Here's the drawing with two shaded views (mm, measured from the low corner). I have some questions. Coordinates: 2 decimals unless noted, no trailing zeros. Write each loop counter-clockwise with the first axis right and the second up, starting at its lowest first coordinate (ties: lowest second). Pieces come first, ordered by that corner, then holes. Notation, with made-up numbers: (9, -26.75) -> (23, -26.75) arc R32 ccw to (23, 3.25) -> close; hole circle Ø11 at (51.25, -22.5). An arc over 180 degrees is marked (long way). Put each result on its own line as item: value. Start each with the question number.
Item 1: I want a section at B-B, the plane y = 8.5. List the corners of the cut face in (x, z) for me.
Item 2: I want a section at C-C, the plane z = 1.5. List the corners of the cut face in (x, y) for me.
Item 3: I need wall thicknesses on line 1 (X direction, y = 9, z = 1.2); line 2 (Y direction, x = 35, z = 1.45); line 3 (Y direction, x = 14, z = 0.25). Which ranges of each line are inside material? Lowest first, please. Write a range as [from, to].
Item 4: I want a section at A-A, the plane x = 35. List the corners of the cut face in (y, z) for me.
Item 5: I want a section at D-D, the plane x = 24.5. List the corners of the cut face in (y, z) for me, then the cut area to 3 significant figures.
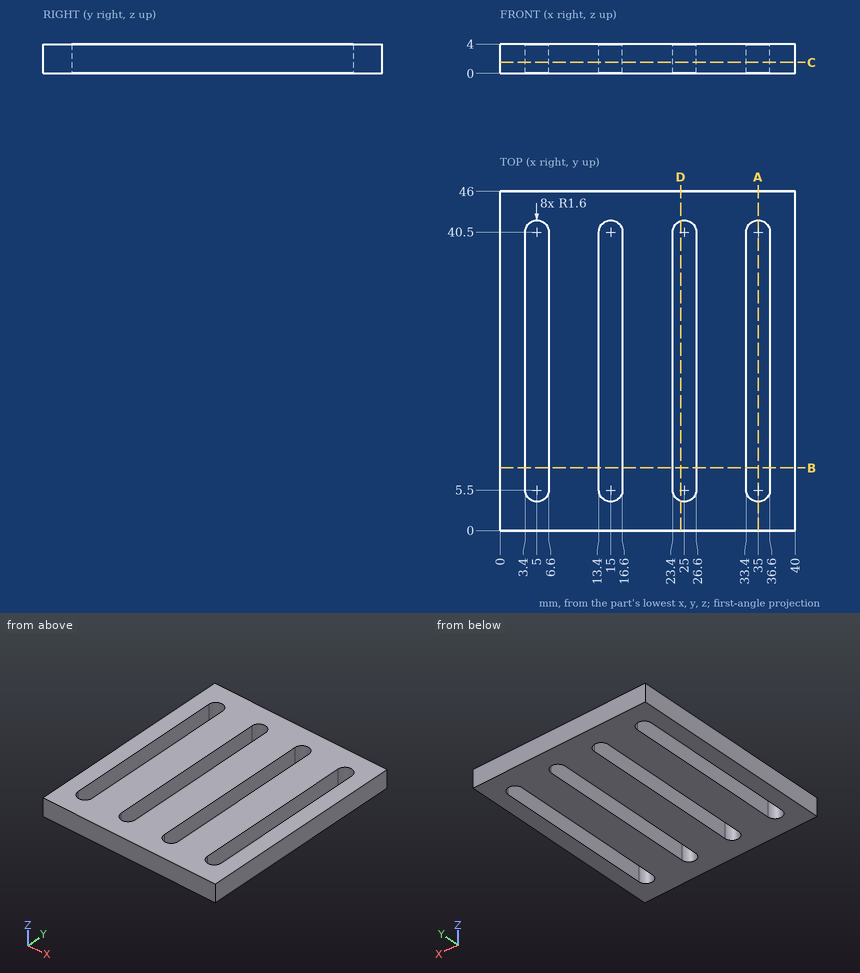
Calculated:
1. outline: (0, 0) -> (3.4, 0) -> (3.4, 4) -> (0, 4) -> close; (6.6, 0) -> (13.4, 0) -> (13.4, 4) -> (6.6, 4) -> close; (16.6, 0) -> (23.4, 0) -> (23.4, 4) -> (16.6, 4) -> close; (26.6, 0) -> (33.4, 0) -> (33.4, 4) -> (26.6, 4) -> close; (36.6, 0) -> (40, 0) -> (40, 4) -> (36.6, 4) -> close
2. outline: (0, 0) -> (40, 0) -> (40, 46) -> (0, 46) -> close; hole (3.4, 5.5) arc R1.6 ccw to (6.6, 5.5) -> (6.6, 40.5) arc R1.6 ccw to (3.4, 40.5) -> close; hole (13.4, 5.5) arc R1.6 ccw to (16.6, 5.5) -> (16.6, 40.5) arc R1.6 ccw to (13.4, 40.5) -> close; hole (23.4, 5.5) arc R1.6 ccw to (26.6, 5.5) -> (26.6, 40.5) arc R1.6 ccw to (23.4, 40.5) -> close; hole (33.4, 5.5) arc R1.6 ccw to (36.6, 5.5) -> (36.6, 40.5) arc R1.6 ccw to (33.4, 40.5) -> close
3. line 1: x = [0, 3.4], [6.6, 13.4], [16.6, 23.4], [26.6, 33.4], [36.6, 40]
3. line 2: y = [0, 3.9], [42.1, 46]
3. line 3: y = [0, 4.25], [41.75, 46]
4. outline: (0, 0) -> (3.9, 0) -> (3.9, 4) -> (0, 4) -> close; (42.1, 0) -> (46, 0) -> (46, 4) -> (42.1, 4) -> close
5. outline: (0, 0) -> (3.98, 0) -> (3.98, 4) -> (0, 4) -> close; (42.02, 0) -> (46, 0) -> (46, 4) -> (42.02, 4) -> close
5. area: 31.8 mm2
